Here's how the part is built. I have some questions about the finished solid (model axes, mm). Face numbers are marked on the shaded views. A direction names the side the tool comes from. Round coordinates to 2 decimals unless told otherwise and drop trailing zeros. Loops run counter-clockwise (first coordinate to the right, second up) from the corner with the lowest first, then second, coordinate; pieces in that order, holes last. Notation, with made-up numbers: M 50,72 L 73,72 A13 cw 73,91 Z; hole C -25,77.5 d4. An arc over 180 degrees is marked long. Answer as CSV lines item,"result".
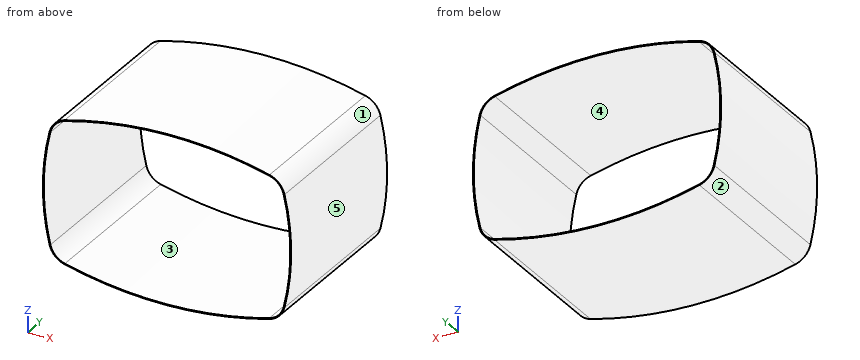
```python
from build123d import *

# Parameters (mm, degrees)
BOSS_EXTRUDE1_DEPTH = 200
SHELL3_T            = -1
CUT_EXTRUDE1_DEPTH  = 200


with BuildPart() as part:
    # Sketch1 → Boss-Extrude1 (new body)
    with BuildSketch(Plane(origin=(0, 0, 0), x_dir=(1, 0, 0), z_dir=(0, 1, 0))):
        with BuildLine():
            ThreePointArc((-121.409753109, 84.164334567), (-132.846711046, 77.506995883), (-139.283044385, 65.944220336))
            ThreePointArc((-139.283044385, 65.944220336), (-147.236834181, 0), (-139.283044385, -65.944220336))
            ThreePointArc((-139.283044385, -65.944220336), (-132.846711046, -77.506995883), (-121.409753109, -84.164334567))
            ThreePointArc((-121.409753109, -84.164334567), (0, -99.99301504), (121.409753109, -84.164334567))
            ThreePointArc((121.409753109, -84.164334567), (132.846711046, -77.506995883), (139.283044385, -65.944220336))
            ThreePointArc((139.283044385, -65.944220336), (147.236834181, 0), (139.283044385, 65.944220336))
            ThreePointArc((139.283044385, 65.944220336), (132.846711046, 77.506995883), (121.409753109, 84.164334567))
            ThreePointArc((121.409753109, 84.164334567), (0, 99.99301504), (-121.409753109, 84.164334567))
        make_face()
    extrude(amount=BOSS_EXTRUDE1_DEPTH)

    # Shell3
    shell3_openings = [part.faces().sort_by_distance(p)[0] for p in [
        (0, 200, 0),
    ]]
    offset(amount=SHELL3_T, openings=shell3_openings, kind=Kind.INTERSECTION)

    # Sketch3 → Cut-Extrude1 (cut)
    with BuildSketch(Plane.XZ):
        with BuildLine():
            ThreePointArc((-121.153362985, -83.197761185), (0, -98.99301504), (121.153362985, -83.197761185))
            ThreePointArc((121.153362985, -83.197761185), (132.132842604, -76.806716048), (138.311722609, -65.706451522))
            ThreePointArc((138.311722609, -65.706451522), (146.236834181, 0), (138.311722609, 65.706451522))
            ThreePointArc((138.311722609, 65.706451522), (132.132842604, 76.806716048), (121.153362985, 83.197761185))
            ThreePointArc((121.153362985, 83.197761185), (0, 98.99301504), (-121.153362985, 83.197761185))
            ThreePointArc((-121.153362985, 83.197761185), (-132.132842604, 76.806716048), (-138.311722609, 65.706451522))
            ThreePointArc((-138.311722609, 65.706451522), (-146.236834181, 0), (-138.311722609, -65.706451522))
            ThreePointArc((-138.311722609, -65.706451522), (-132.132842604, -76.806716048), (-121.153362985, -83.197761185))
        make_face()
    extrude(amount=-CUT_EXTRUDE1_DEPTH, mode=Mode.SUBTRACT)


solid = part.part
```
1. We'd pull the mould along X, two halves only. Please class the marked faces 1, 2 and 3: pulls with the +X half, pulls with the -X half, needs draft (parallel to the pull), parting line crosses it, or undercut.
Evaluation:
face 1,"pulls with the +X half"
face 2,"pulls with the -X half"
face 3,"undercut"
2. I want a section at C-C, the plane z = 29. Please give me the cut outline in (x, y), and give its area (3 significant figures).
Evaluation:
outline,"M -145.72,0 L -144.71,0 L -144.71,200 L -145.72,200 Z; M 144.71,0 L 145.72,0 L 145.72,200 L 144.71,200 Z"
area,"402 mm²"
3. I want a section at A-A, the plane y = 116. Please give me the cut outline in (x, z).
Evaluation:
outline,"M -139.28,-65.94 A25 ccw -121.41,-84.16 A473.54 ccw 121.41,-84.16 A25 ccw 139.28,-65.94 A277.35 ccw 139.28,65.94 A25 ccw 121.41,84.16 A473.54 ccw -121.41,84.16 A25 ccw -139.28,65.94 A277.35 ccw Z; hole M -138.31,-65.71 A24 ccw -121.15,-83.2 A472.54 ccw 121.15,-83.2 A24 ccw 138.31,-65.71 A276.35 ccw 138.31,65.71 A24 ccw 121.15,83.2 A472.54 ccw -121.15,83.2 A24 ccw -138.31,65.71 A276.35 ccw Z"
4. If I drill on line 1 (X direction, y = 135, z = 23.5); line 2 (Z direction, x = 56, y = 98.5); line 3 (Z direction, x = 66, y = 163.5), over which ranges is the centre line in solid material (lowest first)? Write a range as [from, to].
Evaluation:
line 1,"x = [-146.24, -145.24], [145.24, 146.24]"
line 2,"z = [-96.67, -95.66], [95.66, 96.67]"
line 3,"z = [-95.37, -94.36], [94.36, 95.37]"
5. Which directions (+Z, -Z, +X, -X, +Y, -Y) give clear straight access to the entire face, cutting with the end or side of a thin tool? Please do the marked faces 4 and 5.
Evaluation:
face 4,"+Y, -Y"
face 5,"+X, +Y, -Y"
6. I want a section at B-B, the plane x = -26.5. Please give me the cut outline in (y, z), and give its area (3 significant figures).
Evaluation:
outline,"M 0,-99.25 L 200,-99.25 L 200,-98.25 L 0,-98.25 Z; M 0,98.25 L 200,98.25 L 200,99.25 L 0,99.25 Z"
area,"401 mm²"
7. For P1, Ø8, axis at x = -107, y = 174.5, coming from the +Z side; P2, Ø5, axis at y = 113, z = -24, coming from the -X side; P3, Ø12, axis at y = 41.5, z = -79.5, coming from the +X side, each with a flat end and sliding along its axis, tell me the tip position at first contact or that it passes through.
Evaluation:
P1,"stops at z = 88.66"
P2,"stops at x = -146.4"
P3,"stops at x = 136.04"
